Job drawing, mm, ordinate dimensions from the low corner. One solid piece. A direction names the side the tool comes from. Coordinates: 2 decimals unless noted, no trailing zeros. Loops run counter-clockwise (first coordinate to the right, second up) from the corner with the lowest first, then second, coordinate; pieces in that order, holes last. Notation, with made-up numbers: (24.25, 28.5) - (63.25, 28.5) arc R13 ccw to (63.25, 44.5) - close; hole circle Ø8 at (31, 87). An arc over 180 degrees is marked (long way). Use a Markdown table: item, result. Add a question column.
1) Band-saw the part on B-B (y = 47). Give the cut face in (x, z) (1 decimal), plus the area to 3 significant figures.
2) Tool access for the marked faces 3, 4 and 5: list every direction of +Z, -Z, +X, -X, +Y, -Y with a clear straight run to the whole face (end or side of a thin tool).
3) Band-saw the part on D-D (x = 20.5). Give the cut face in (y, z) (1 decimal).
4) Band-saw the part on A-A (x = 42.5). Give the cut face in (y, z), plus the area to 3 significant figures.
5) Drop flat-ended pins along their axis: P1, Ø1.5, axis at x = 35, y = 34, coming from the -Z side; P2, Ø3, axis at x = 46, y = 21, coming from the +Z side; P3, Ø8, axis at x = 59.5, z = 14.5, coming from the -Y side; P4, Ø5, axis at x = 69.5, y = 25.5, coming from the +Z side. Give the stop position or say it passes through.
6) Pull direction X, two halves, no side cores. Call the marked faces 1 and 2: +X half, -X half, draft (parallel to the pull), parting line (faces both ways), or undercut.
7) Band-saw the part on C-C (z = 46). Give the cut face in (x, y), plus the area to 3 significant figures.
8) Probe probe 1 along Z at (x, y) = (9.5, 42.5); probe 2 along Z at (x, y) = (17.5, 56); probe 3 along Y at (x, z) = (7, 40.5) (1 decimal). List the from-to ranges inside material, lowest first. Write a range as [from, to].
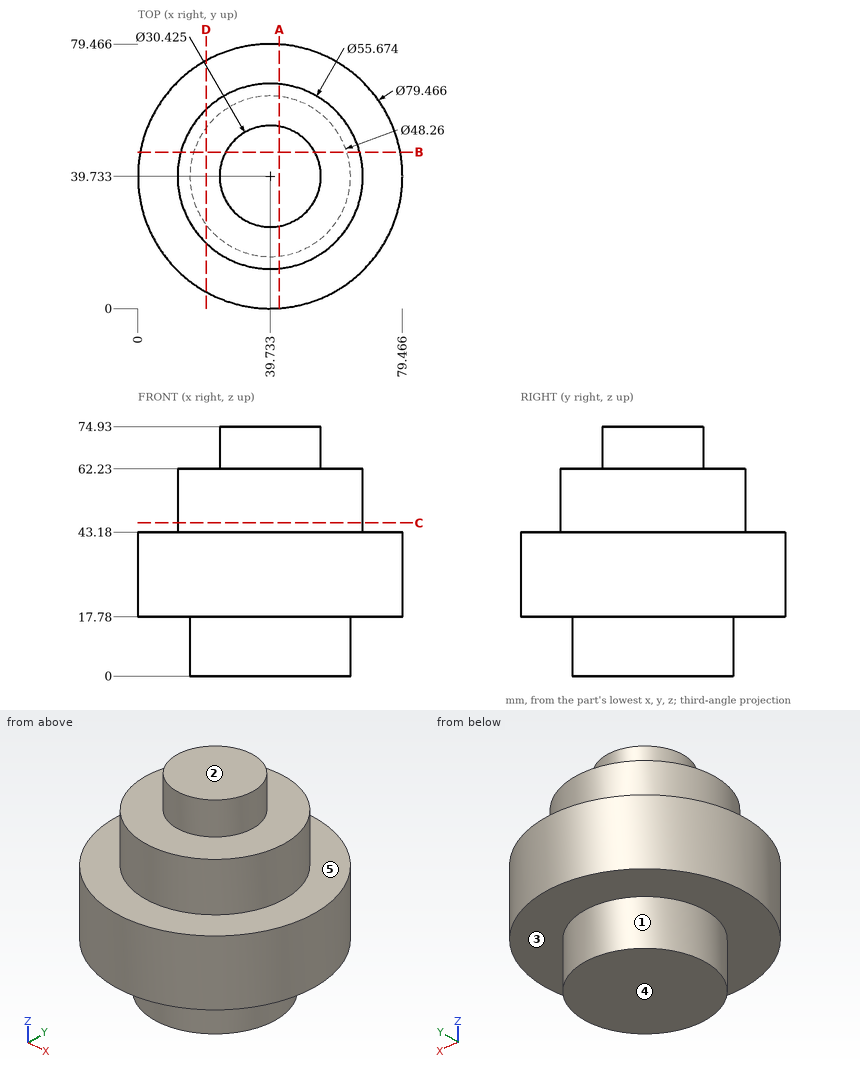
Answer block:
| question | item | result |
|---|---|---|
| 1 | outline | (0.7, 17.8) - (16.7, 17.8) - (16.7, 0) - (62.7, 0) - (62.7, 17.8) - (78.8, 17.8) - (78.8, 43.2) - (66.6, 43.2) - (66.6, 62.2) - (53.1, 62.2) - (53.1, 74.9) - (26.4, 74.9) - (26.4, 62.2) - (12.9, 62.2) - (12.9, 43.2) - (0.7, 43.2) - close |
| 1 | area | 4,170 mm2 |
| 2 | face 3 | -Z |
| 2 | face 4 | -Z, +X, -X, +Y, -Y |
| 2 | face 5 | +Z |
| 3 | outline | (5, 17.8) - (25.2, 17.8) - (25.2, 0) - (54.3, 0) - (54.3, 17.8) - (74.5, 17.8) - (74.5, 43.2) - (59.9, 43.2) - (59.9, 62.2) - (19.6, 62.2) - (19.6, 43.2) - (5, 43.2) - close |
| 4 | outline | (0.1, 17.78) - (15.76, 17.78) - (15.76, 0) - (63.7, 0) - (63.7, 17.78) - (79.37, 17.78) - (79.37, 43.18) - (67.43, 43.18) - (67.43, 62.23) - (54.69, 62.23) - (54.69, 74.93) - (24.77, 74.93) - (24.77, 62.23) - (12.03, 62.23) - (12.03, 43.18) - (0.1, 43.18) - close |
| 4 | area | 4,300 mm2 |
| 5 | P1 | z = 0 |
| 5 | P2 | z = 62.23 |
| 5 | P3 | y = 4.05 |
| 5 | P4 | z = 43.18 |
| 6 | face 1 | parting line |
| 6 | face 2 | draft |
| 7 | outline | circle Ø55.67 at (39.73, 39.73) |
| 7 | area | 2,430 mm2 |
| 8 | probe 1 | [17.78, 43.18] |
| 8 | probe 2 | [17.78, 62.23] |
| 8 | probe 3 | [17.2, 62.3] |
